Read the model definition and answer for the solid it produces. Units are mm, in the model's axes. Face numbers are marked on the shaded views. Round coordinates to 2 decimals unless told otherwise and drop trailing zeros. Loops run counter-clockwise (first coordinate to the right, second up) from the corner with the lowest first, then second, coordinate; pieces in that order, holes last. Notation, with made-up numbers: (20, 30) -> (73, 30) arc R18 ccw to (73, 39) -> close; hole circle Ø3 at (32, 37.5). An arc over 180 degrees is marked (long way). Put each result on its own line as item: value.
from build123d import *

# Parameters (mm, degrees)
SKETCH1_W           = 56
SKETCH1_H           = 4
SKETCH1_R           = 1.25
SKETCH1_R_2         = 1.15
BOSS_EXTRUDE1_DEPTH = 5
FILLET1_R           = 2
SKETCH2_R           = 2
SKETCH2_R_2         = 1.25
BOSS_EXTRUDE2_DEPTH = 2


with BuildPart() as part:
    # Sketch1 → Boss-Extrude1 (new body)
    with BuildSketch(Plane(origin=(0, 0, 0), x_dir=(1, 0, 0), z_dir=(0, 1, 0))):
        with Locations((28, 2)):
            Rectangle(SKETCH1_W, SKETCH1_H)
        with Locations(Location((2, 2, 0), (0, 0, 270))):
            Circle(SKETCH1_R, mode=Mode.SUBTRACT)
        with Locations(Location((16.5, 2, 0), (0, 0, 270))):
            Circle(SKETCH1_R_2, mode=Mode.SUBTRACT)
        with Locations(Location((23.5, 2, 0), (0, 0, 270))):
            Circle(SKETCH1_R_2, mode=Mode.SUBTRACT)
        with Locations(Location((54, 2, 0), (0, 0, 90))):
            Circle(SKETCH1_R, mode=Mode.SUBTRACT)
        with Locations(Location((30.5, 2, 0), (0, 0, 90))):
            Circle(SKETCH1_R_2, mode=Mode.SUBTRACT)
        with Locations(Location((37.5, 2, 0), (0, 0, 90))):
            Circle(SKETCH1_R_2, mode=Mode.SUBTRACT)
    extrude(amount=BOSS_EXTRUDE1_DEPTH)

    # Fillet1
    fillet1_edges = [part.edges().sort_by_distance(p)[0] for p in [
        (56, 2.5, -4),
        (56, 2.5, 0),
        (0, 2.5, -4),
        (0, 2.5, 0),
    ]]
    fillet(fillet1_edges, radius=FILLET1_R - 0.0001)  # a hair under: the kernel refuses the full size

    # Sketch2 → Boss-Extrude2 (add)
    # profile 1 of 2: a face of its own
    with BuildSketch(Plane(origin=(0, 5, 0), x_dir=(1, 0, 0), z_dir=(0, 1, 0))):
        with Locations(Location((2, 2, 0), (0, 0, 270))):
            Circle(SKETCH2_R)
        with Locations(Location((2, 2, 0), (0, 0, 270))):
            Circle(SKETCH2_R_2, mode=Mode.SUBTRACT)
    # profile 2 of 2: a face of its own
    with BuildSketch(Plane(origin=(0, 5, 0), x_dir=(1, 0, 0), z_dir=(0, 1, 0))):
        with Locations(Location((54, 2, 0), (0, 0, 270))):
            Circle(SKETCH2_R)
        with Locations(Location((54, 2, 0), (0, 0, 90))):
            Circle(SKETCH2_R_2, mode=Mode.SUBTRACT)
    extrude(amount=BOSS_EXTRUDE2_DEPTH)


solid = part.part
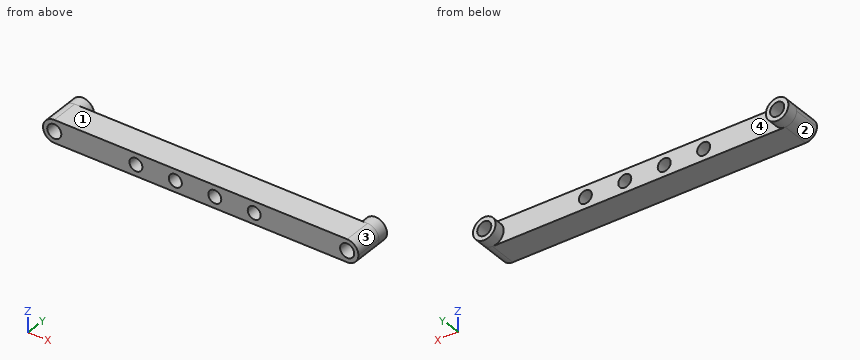
Item 1: Find the intervals of material crossed by line 1 along Z through (x, y) = (54, 5.75); line 2 along X through (y, z) = (5.5, -2); line 3 along Z through (x, y) = (37.5, 2.6), in increasing order.
Derived:
line 1: z = -4 to -3.25, -0.75 to 0
line 2: x = 0 to 0.75, 3.25 to 4, 52 to 52.75, 55.25 to 56
line 3: z = -4 to -3.15, -0.85 to 0
Item 2: The part is cut by section C-C (x = 25.5). Determine the outline of the cut face in (y, z), then the cut area to 3 significant figures.
Derived:
outline: (0, -4) -> (5, -4) -> (5, 0) -> (0, 0) -> close
area: 20.0 mm^2
Item 3: The part is cut by section B-B (y = 4). State how many separate pieces and enclosed holes the cut face has, then the cut area to 3 significant figures.
Derived:
separate pieces: 1
enclosed holes: 6
area: 194 mm^2
Item 4: The part is cut by section A-A (x = 37.5). Determine the outline of the cut face in (y, z), then the cut area to 3 significant figures.
Derived:
outline: (0, -4) -> (5, -4) -> (5, -3.15) -> (0, -3.15) -> close; (0, -0.85) -> (5, -0.85) -> (5, 0) -> (0, 0) -> close
area: 8.50 mm^2
Item 5: For a pull along X with two mould halves and no side action, classify the marked faces 1, 2, 3 and 4 as pulls with the +X half, pulls with the -X half, needs draft (parallel to the pull), parting line crosses it, or undercut.
Derived:
face 1: needs draft
face 2: pulls with the -X half
face 3: pulls with the +X half
face 4: undercut
